```python
from build123d import *

# Parameters (mm, degrees)
SKETCH1_W           = 19.05
SKETCH1_H           = 50.8
SKETCH1_W_2         = 76.2
SKETCH1_H_2         = 76.2
BOSS_EXTRUDE1_DEPTH = 25.4


with BuildPart() as part:
    # Sketch1 → Boss-Extrude1 (new body)
    with BuildSketch(Plane.XY):
        Polygon((0, 0), (0, 50.8), (57.15, 88.9), (158.75, 88.9), (215.9, 50.8), (215.9, 0), (158.75, -38.1), (57.15, -38.1), align=None)
        with Locations((34.925, 25.4)):
            Rectangle(SKETCH1_W, SKETCH1_H, mode=Mode.SUBTRACT)
        with Locations((107.95, 23.124358826)):
            Rectangle(SKETCH1_W_2, SKETCH1_H_2, mode=Mode.SUBTRACT)
        with Locations((180.975, 25.4)):
            Rectangle(SKETCH1_W, SKETCH1_H, mode=Mode.SUBTRACT)
    extrude(amount=BOSS_EXTRUDE1_DEPTH)


solid = part.part
```
Input: part model. Units: mm. Frame: model coordinates. A direction names the side the tool comes from. Give positions to 0.01 mm unless a question says otherwise; leave off trailing zeros. Order: outer loops, then holes, each group sorted by start corner. A loop starts at its lowest first (then second) coordinate and runs counter-clockwise, first axis right, second up. Notation, with made-up numbers: (29.5, 5) - (71.5, 5) arc R16 ccw to (71.5, 9) - close; hole circle Ø7 at (61.5, 59). An arc over 180 degrees is marked (long way). Put each result on its own line as item: value.
Item 1: Draft query along Y for faces 3 (the flat face through (109, -16, 25.4)), 4 (the flat face through (107, 88.9, 13)), 5 (the flat face through (171.45, 25, 13)). Return one class per face: +Y half, -Y half, draft (parallel to the pull), parting line (faces both ways), or undercut.
Found:
face 3: draft
face 4: +Y half
face 5: undercut
Item 2: Access query for faces 1 (the flat face through (215.9, 26, 13)), 2 (the flat face through (181, 50.8, 13)). Directions: +Z, -Z, +X, -X, +Y, -Y. A direction counts if a zero-diameter tool reaches every point of the face in a straight line with its end or side. Return the directions, or none.
Found:
face 1: +Z, -Z, +X, +Y, -Y
face 2: +Z, -Z
Item 3: Section query D-D, the plane y = 35. Return loops of the section in (x, z), then the cut area to 3 significant figures.
Found:
outline: (0, 0) - (25.4, 0) - (25.4, 25.4) - (0, 25.4) - close; (44.45, 0) - (69.85, 0) - (69.85, 25.4) - (44.45, 25.4) - close; (146.05, 0) - (171.45, 0) - (171.45, 25.4) - (146.05, 25.4) - close; (190.5, 0) - (215.9, 0) - (215.9, 25.4) - (190.5, 25.4) - close
area: 2,580 mm^2
Item 4: Contact query for flat-ended pins moving along their axis: pin 1 (1 mm diameter, centred on x = 33.5, y = -11, fed in from -Z); pin 2 (15 mm diameter, centred on x = 184, z = 15, fed in from -Y); pin 3 (5.5 mm diameter, centred on x = 38.5, z = 6.5, fed in from -Y); pin 4 (4 mm diameter, centred on y = -8, z = 14.5, fed in from -X). Output: stop coordinate, or through.
Found:
pin 1: stops at z = 0
pin 2: stops at y = -26.27
pin 3: stops at y = -27.5
pin 4: stops at x = 9
Item 5: Section query B-B, the plane y = 54. Return loops of the section in (x, z).
Found:
outline: (4.8, 0) - (69.85, 0) - (69.85, 25.4) - (4.8, 25.4) - close; (146.05, 0) - (211.1, 0) - (211.1, 25.4) - (146.05, 25.4) - close
Item 6: Section query C-C, the plane z = 11.75. Return loops of the section in (x, y), then the cut area to 3 significant figures.
Found:
outline: (0, 0) - (57.15, -38.1) - (158.75, -38.1) - (215.9, 0) - (215.9, 50.8) - (158.75, 88.9) - (57.15, 88.9) - (0, 50.8) - close; hole (25.4, 0) - (44.45, 0) - (44.45, 50.8) - (25.4, 50.8) - close; hole (69.85, -14.98) - (146.05, -14.98) - (146.05, 61.22) - (69.85, 61.22) - close; hole (171.45, 0) - (190.5, 0) - (190.5, 50.8) - (171.45, 50.8) - close
area: 15,300 mm^2
Item 7: Section query A-A, the plane x = 104.5. Return loops of the section in (y, z).
Found:
outline: (-38.1, 0) - (-14.98, 0) - (-14.98, 25.4) - (-38.1, 25.4) - close; (61.22, 0) - (88.9, 0) - (88.9, 25.4) - (61.22, 25.4) - close
Item 8: Ray query, L1, parallel to X at y = 25, z = 13; L2, parallel to Y at x = 124.5, z = 9.5; L3, parallel to Y at x = 26.5, z = 20.75. Return the intervals inside material, ascending. Write a range as from..to.
Found:
L1: x = 0..25.4, 44.45..69.85, 146.05..171.45, 190.5..215.9
L2: y = -38.1..-14.98, 61.22..88.9
L3: y = -17.67..0, 50.8..68.47
